Geometry check sheet. Reference: the model listing, model coordinates, mm. Round coordinates to 2 decimals unless told otherwise and drop trailing zeros.
from build123d import *

# Parameters (mm, degrees)
EXTRUDE_1_OUTLINE_R   = 100
EXTRUDE_1_OUTLINE_R_2 = 2
EXTRUDE_1_DEPTH       = 3
CUT_EXTRUDE_1_DEPTH   = 30
SKETCH_6_R            = 1.5
SKETCH_6_R_2          = 2
CUT_EXTRUDE_2_DEPTH   = 10
CUT_EXTRUDE_4_DEPTH   = 10
SKETCH_9_R            = 1.5
CUT_EXTRUDE_5_DEPTH   = 10


# Read off the part's stored shape, not the designer's step: 填料-伸長1
with BuildPart() as part:
    # 填料-伸長1 outline → 填料-伸長1 (new body)
    with BuildSketch(Plane.XY):
        Circle(EXTRUDE_1_OUTLINE_R)
        with Locations((-60, -55)):
            Circle(EXTRUDE_1_OUTLINE_R_2, mode=Mode.SUBTRACT)
        with Locations((60, -55)):
            Circle(EXTRUDE_1_OUTLINE_R_2, mode=Mode.SUBTRACT)
        with Locations((-60, 55)):
            Circle(EXTRUDE_1_OUTLINE_R_2, mode=Mode.SUBTRACT)
        with Locations((60, 55)):
            Circle(EXTRUDE_1_OUTLINE_R_2, mode=Mode.SUBTRACT)
    extrude(amount=EXTRUDE_1_DEPTH)

    # 草圖5 → 除料-伸長1 (cut)
    with BuildSketch(Plane.XY.offset(3)):
        with BuildLine():
            Line((68.5, -40), (71.5, -40))
            ThreePointArc((71.5, -40), (72.207106781, -39.707106781), (72.5, -39))
            Line((72.5, -39), (72.5, 39))
            ThreePointArc((72.5, 39), (72.207106781, 39.707106781), (71.5, 40))
            Line((71.5, 40), (68.5, 40))
            ThreePointArc((68.5, 40), (67.792893219, 39.707106781), (67.5, 39))
            Line((67.5, 39), (67.5, -39))
            ThreePointArc((67.5, -39), (67.792893219, -39.707106781), (68.5, -40))
        make_face()
    extrude(amount=-CUT_EXTRUDE_1_DEPTH, mode=Mode.SUBTRACT)

    # 草圖6 → 除料-伸長2 (cut)
    with BuildSketch(Plane.XY.offset(3)):
        with Locations((-63.405422156, 35.137513831)):
            Circle(SKETCH_6_R)
        with Locations((-14.405422156, 35.137513831)):
            Circle(SKETCH_6_R)
        with Locations((-14.405422156, -22.862486169)):
            Circle(SKETCH_6_R)
        with Locations((-63.405422156, -22.862486169)):
            Circle(SKETCH_6_R)
        with Locations((41.73785257, 33.212145781)):
            Circle(SKETCH_6_R)
        with Locations((13.79785257, 33.212145781)):
            Circle(SKETCH_6_R)
        with Locations((-1.44214743, -16.317854219)):
            Circle(SKETCH_6_R)
        with Locations((46.81785257, -17.587854219)):
            Circle(SKETCH_6_R)
        with Locations((-22.75, 62.76204956)):
            Circle(SKETCH_6_R)
        with Locations((22.75, 62.76204956)):
            Circle(SKETCH_6_R)
        with Locations((59, 17)):
            Circle(SKETCH_6_R)
        with Locations((59, -17)):
            Circle(SKETCH_6_R)
        with Locations((81, -17)):
            Circle(SKETCH_6_R)
        with Locations((81, 17)):
            Circle(SKETCH_6_R)
        with Locations((-90, 20)):
            Circle(SKETCH_6_R_2)
        with Locations((-90, -20)):
            Circle(SKETCH_6_R_2)
        with Locations((-75, 20)):
            Circle(SKETCH_6_R_2)
        with Locations((-75, -20)):
            Circle(SKETCH_6_R_2)
    extrude(amount=-CUT_EXTRUDE_2_DEPTH, mode=Mode.SUBTRACT)

    # 草圖8 → 除料-伸長4 (cut)
    with BuildSketch(Plane.XY.offset(3)):
        with BuildLine():
            Line((-42.5, -48.5), (-37.5, -48.5))
            ThreePointArc((-37.5, -48.5), (-36, -50), (-37.5, -51.5))
            Line((-37.5, -51.5), (-42.5, -51.5))
            ThreePointArc((-42.5, -51.5), (-44, -50), (-42.5, -48.5))
        make_face()
        with BuildLine():
            Line((-22.5, -51.5), (-17.5, -51.5))
            ThreePointArc((-17.5, -51.5), (-16, -50), (-17.5, -48.5))
            Line((-17.5, -48.5), (-22.5, -48.5))
            ThreePointArc((-22.5, -48.5), (-24, -50), (-22.5, -51.5))
        make_face()
        with BuildLine():
            Line((-2.5, -51.5), (2.5, -51.5))
            ThreePointArc((2.5, -51.5), (4, -50), (2.5, -48.5))
            Line((2.5, -48.5), (-2.5, -48.5))
            ThreePointArc((-2.5, -48.5), (-4, -50), (-2.5, -51.5))
        make_face()
        with BuildLine():
            Line((17.5, -51.5), (22.5, -51.5))
            ThreePointArc((22.5, -51.5), (24, -50), (22.5, -48.5))
            Line((22.5, -48.5), (17.5, -48.5))
            ThreePointArc((17.5, -48.5), (16, -50), (17.5, -51.5))
        make_face()
        with BuildLine():
            Line((37.5, -51.5), (42.5, -51.5))
            ThreePointArc((42.5, -51.5), (44, -50), (42.5, -48.5))
            Line((42.5, -48.5), (37.5, -48.5))
            ThreePointArc((37.5, -48.5), (36, -50), (37.5, -51.5))
        make_face()
        with BuildLine():
            Line((-42.5, -68.5), (-37.5, -68.5))
            ThreePointArc((-37.5, -68.5), (-36, -70), (-37.5, -71.5))
            Line((-37.5, -71.5), (-42.5, -71.5))
            ThreePointArc((-42.5, -71.5), (-44, -70), (-42.5, -68.5))
        make_face()
        with BuildLine():
            Line((-22.5, -68.5), (-17.5, -68.5))
            ThreePointArc((-17.5, -68.5), (-16, -70), (-17.5, -71.5))
            Line((-17.5, -71.5), (-22.5, -71.5))
            ThreePointArc((-22.5, -71.5), (-24, -70), (-22.5, -68.5))
        make_face()
        with BuildLine():
            Line((-2.5, -68.5), (2.5, -68.5))
            ThreePointArc((2.5, -68.5), (4, -70), (2.5, -71.5))
            Line((2.5, -71.5), (-2.5, -71.5))
            ThreePointArc((-2.5, -71.5), (-4, -70), (-2.5, -68.5))
        make_face()
        with BuildLine():
            Line((17.5, -68.5), (22.5, -68.5))
            ThreePointArc((22.5, -68.5), (24, -70), (22.5, -71.5))
            Line((22.5, -71.5), (17.5, -71.5))
            ThreePointArc((17.5, -71.5), (16, -70), (17.5, -68.5))
        make_face()
        with BuildLine():
            Line((37.5, -68.5), (42.5, -68.5))
            ThreePointArc((42.5, -68.5), (44, -70), (42.5, -71.5))
            Line((42.5, -71.5), (37.5, -71.5))
            ThreePointArc((37.5, -71.5), (36, -70), (37.5, -68.5))
        make_face()
    extrude(amount=-CUT_EXTRUDE_4_DEPTH, mode=Mode.SUBTRACT)

    # 草圖9 → 除料-伸長5 (cut)
    with BuildSketch(Plane.XY.offset(3)):
        with Locations((95, 0)):
            Circle(SKETCH_9_R)
        with Locations((79.919085619, -51.360877658)):
            Circle(SKETCH_9_R)
        with Locations((39.464426235, -86.415039559)):
            Circle(SKETCH_9_R)
        with Locations((-13.519909636, -94.033036979)):
            Circle(SKETCH_9_R)
        with Locations((-62.211769725, -71.796209564)):
            Circle(SKETCH_9_R)
        with Locations((-91.151832493, -26.7645929)):
            Circle(SKETCH_9_R)
        with Locations((-91.151832493, 26.7645929)):
            Circle(SKETCH_9_R)
        with Locations((-62.211769725, 71.796209564)):
            Circle(SKETCH_9_R)
        with Locations((-13.519909636, 94.033036979)):
            Circle(SKETCH_9_R)
        with Locations((39.464426235, 86.415039559)):
            Circle(SKETCH_9_R)
        with Locations((79.919085619, 51.360877658)):
            Circle(SKETCH_9_R)
    extrude(amount=-CUT_EXTRUDE_5_DEPTH, mode=Mode.SUBTRACT)


solid = part.part
1. Scan lines: line 1 along Y through (x, z) = (-38, 0.7); line 2 along Y through (x, z) = (-40, 1.7); line 3 along X through (y, z) = (-69.5, 0.45). Record each from-to range of solid material in increasing order.
2. Section check A-A (z = 2.3). State how many separate pieces and enclosed holes the cut face has, plus the area to 3 significant figures.
3. Depth check by flat-ended pin: pin 1 Ø5 at (x, y) = (95, 0) entering from +Z; pin 2 Ø0.9 at (x, z) = (40, 1) entering from +Y; pin 3 Ø1.5 at (y, z) = (-13.5, 1) entering from +X; pin 4 Ø1.5 at (x, z) = (-39, 1) entering from +Y. Enter the tip coordinate at first touch or a pass-through.
Results below:
1. line 1: y = -92.5 to -71.5, -68.5 to -51.5, -48.5 to 92.5
1. line 2: y = -91.65 to -71.5, -68.5 to -51.5, -48.5 to 91.65
1. line 3: x = -71.9 to -43.91, -36.09 to -23.91, -16.09 to -3.91, 3.91 to 16.09, 23.91 to 36.09, 43.91 to 71.9
2. separate pieces: 1
2. enclosed holes: 44
2. area: 30,500 mm2
3. pin 1: stops at z = 3
3. pin 2: stops at y = 91.85
3. pin 3: stops at x = 99.18
3. pin 4: stops at y = 92.4
